Source: CAD feature listing. Evaluate the final solid. Frame: model axes, mm. A direction names the side the tool comes from. Round coordinates to 2 decimals unless told otherwise and drop trailing zeros. Loops run counter-clockwise (first coordinate to the right, second up) from the corner with the lowest first, then second, coordinate; pieces in that order, holes last. Notation, with made-up numbers: M 68,-31 L 82,-31 A23 ccw 82,7 Z; hole C 33,10.25 d2. An arc over 180 degrees is marked long. One line per item, written item: value.
from build123d import *

# Parameters (mm, degrees)
F0_W     = 15
F0_H     = 20
F0_R     = 1.25
F0_R_2   = 1.4668994292
F1_DEPTH = 5
F2_W     = 40
F2_H     = 40
F2_R     = 1.5
F2_W_2   = 15
F2_H_2   = 20
F2_R_2   = 1.25
F3_DEPTH = 10
F4_R     = 2.5


with BuildPart() as f1:
    # F0 (on Front) → F1 (new body)
    with BuildSketch(Plane.XZ):
        with Locations((2.2486895237, 35.21458745)):
            Rectangle(F0_W, F0_H)
        with BuildLine():
            ThreePointArc((2.2486895237, 31.46458745), (3.1325730002, 31.0984709265), (3.4986895237, 30.21458745))
            ThreePointArc((3.4986895237, 30.21458745), (1.3648060472, 29.3307039735), (2.2486895237, 31.46458745))
        make_face(mode=Mode.SUBTRACT)
        with Locations((-2.2513104763, 40.21458745)):
            Circle(F0_R, mode=Mode.SUBTRACT)
        with Locations((6.7486895237, 40.21458745)):
            Circle(F0_R_2, mode=Mode.SUBTRACT)
    extrude(amount=F1_DEPTH)

    # F2 (on face) → F3 (join)
    with BuildSketch(Plane.XZ.offset(5)):
        with Locations((2.2486895237, 35.21458745)):
            Rectangle(F2_W, F2_H)
        with Locations((-13.7513104763, 19.21458745)):
            Circle(F2_R, mode=Mode.SUBTRACT)
        with Locations((2.2486895237, 35.21458745)):
            Rectangle(F2_W_2, F2_H_2, mode=Mode.SUBTRACT)
        with Locations((18.2486895237, 19.21458745)):
            Circle(F2_R, mode=Mode.SUBTRACT)
        with Locations((-13.7513104763, 51.21458745)):
            Circle(F2_R, mode=Mode.SUBTRACT)
        with Locations((18.2486895237, 51.21458745)):
            Circle(F2_R, mode=Mode.SUBTRACT)
        with BuildLine():
            Line((9.7486895237, 25.21458745), (9.7486895237, 45.21458745))
            Line((9.7486895237, 45.21458745), (7.0718369676, 41.6454507086))
            ThreePointArc((7.0718369676, 41.6454507086), (7.8945120964, 41.1304938683), (8.2155889529, 40.21458745))
            ThreePointArc((8.2155889529, 40.21458745), (7.1158037309, 38.7943687717), (5.4655420798, 39.5037241914))
            Line((5.4655420798, 39.5037241914), (-5.2513104763, 25.21458745))
            Line((-5.2513104763, 25.21458745), (9.7486895237, 25.21458745))
        make_face()
        with Locations((2.2486895237, 30.21458745)):
            Circle(F2_R_2, mode=Mode.SUBTRACT)
        with BuildLine():
            Line((7.0718369676, 41.6454507086), (9.7486895237, 45.21458745))
            Line((9.7486895237, 45.21458745), (-5.2513104763, 45.21458745))
            Line((-5.2513104763, 45.21458745), (-5.2513104763, 25.21458745))
            Line((-5.2513104763, 25.21458745), (5.4655420798, 39.5037241914))
            ThreePointArc((5.4655420798, 39.5037241914), (5.5751699804, 41.0947271075), (7.0718369676, 41.6454507086))
        make_face()
        with Locations((-2.2513104763, 40.21458745)):
            Circle(F2_R_2, mode=Mode.SUBTRACT)
        with BuildLine():
            ThreePointArc((8.2155889529, 40.21458745), (7.8945120964, 41.1304938683), (7.0718369676, 41.6454507086))
            Line((7.0718369676, 41.6454507086), (5.4655420798, 39.5037241914))
            ThreePointArc((5.4655420798, 39.5037241914), (7.1158037309, 38.7943687717), (8.2155889529, 40.21458745))
        make_face()
        with Locations((-2.2513104763, 40.21458745)):
            Circle(F2_R_2)
        with BuildLine():
            Line((5.4655420798, 39.5037241914), (7.0718369676, 41.6454507086))
            ThreePointArc((7.0718369676, 41.6454507086), (5.5751699804, 41.0947271075), (5.4655420798, 39.5037241914))
        make_face()
        with Locations((2.2486895237, 30.21458745)):
            Circle(F2_R_2)
    extrude(amount=F3_DEPTH)

    # F4
    f4_edges = [f1.edges().sort_by_distance(p)[0] for p in [
        (-5.25131, -5, 35.214587),
        (2.24869, -5, 25.214587),
        (9.74869, -5, 35.214587),
        (2.24869, -5, 45.214587),
    ]]
    fillet(f4_edges, radius=F4_R)


solid = f1.part
1. Section query D-D (x = -4.5). Return the cut outline in (y, z), and give its area (3 significant figures).
Report:
outline: M -15,15.21 L -5,15.21 L -5,22.71 A2.5 cw -2.5,25.21 L 0,25.21 L 0,45.21 L -2.5,45.21 A2.5 cw -5,47.71 L -5,55.21 L -15,55.21 Z
area: 503 mm2
2. Pull-direction query (X, two-part tool) for faces 4 (the face through (9.749, -1, 35)), 5 (the face through (17.06, -9.93, 50.3)), 6 (the face through (-6.003, -4.287, 35.39)), 7 (the face through (2, -10, 15.215)); classes: released by +X, released by -X, zero draft, split by the parting line, or undercut.
Report:
face 4: released by +X
face 5: undercut
face 6: released by -X
face 7: zero draft
3. Section query C-C (z = 28). Return the cut outline in (x, y).
Report:
outline: M -17.75,-15 L 22.25,-15 L 22.25,-5 L 12.25,-5 A2.5 cw 9.75,-2.5 L 9.75,0 L -5.25,0 L -5.25,-2.5 A2.5 cw -7.75,-5 L -17.75,-5 Z
4. Pin query (flat end, axial travel): pin 1 (3 mm diameter, centred on y = -0.5, z = 31.5, fed in from +X); pin 2 (0.8 mm diameter, centred on x = 1.5, y = -1, fed in from -Z); pin 3 (1.5 mm diameter, centred on x = 6.5, z = 20.5, fed in from +Y). Return the tip coordinate at first contact, or that it passes through.
Report:
pin 1: stops at x = 9.75
pin 2: stops at z = 25.21
pin 3: stops at y = -5
5. Reachability of faces 1 (the face through (2, -5, 30)), 2 (the face through (-14.94, -9.93, 18.3)), 3 (the face through (2, -1, 25.215)) from +Z, -Z, +X, -X, +Y, -Y: full face, straight path, thin tool, end or side. Return the list, or none.
Report:
face 1: +Y
face 2: +Y, -Y
face 3: -Z, +X, -X, +Y
6. Ray query, line 1 (Z direction, x = 18, y = -8.75); line 2 (Y direction, x = -11, z = 34); line 3 (X direction, y = -2.75, z = 28.5). Return the intervals inside material, ascending. Write a range as [from, to].
Report:
line 1: z = [15.21, 17.74], [20.69, 49.74], [52.69, 55.21]
line 2: y = [-15, -5]
line 3: x = [-5.26, 9.76]
7. Section query B-B (y = -3). Return the cut outline in (x, z).
Report:
outline: M -5.3,25.16 L 9.8,25.16 L 9.8,45.27 L -5.3,45.27 Z; hole C -2.25,40.21 d2.5; hole C 2.25,30.21 d2.5; hole C 6.75,40.21 d2.93
8. Section query A-A (z = 52). Return the cut outline in (x, y).
Report:
outline: M -17.75,-15 L -15.03,-15 L -15.03,-5 L -17.75,-5 Z; M -12.47,-15 L 16.97,-15 L 16.97,-5 L -12.47,-5 Z; M 19.53,-15 L 22.25,-15 L 22.25,-5 L 19.53,-5 Z
